Can you work these out from the model? Positions are in its coordinate system, mm. A direction names the side the tool comes from. Give positions to 0.01 mm unless a question says otherwise; leave off trailing zeros. Loops run counter-clockwise (first coordinate to the right, second up) from the corner with the lowest first, then second, coordinate; pieces in that order, holes last. Notation, with made-up numbers: (3, 64.25) -> (10, 64.25) arc R16 ccw to (10, 89.25) -> close; hole circle Ø10 at (51, 26). An arc over 180 degrees is marked (long way). Use CSV: the item, a comma, the result in double quotes.
from build123d import *

# Parameters (mm, degrees)
F0_R     = 31
F1_DEPTH = 10


# Not quite as in the source:
# - a feature names something its author has since deleted; it is built from what else it names


with BuildPart() as f1:
    # F0 (on Top) → F1 (new body)
    with BuildSketch(Plane.XY):
        Circle(F0_R)
        with BuildLine():
            ThreePointArc((19.2857142857, 8.310308327), (24.1116779802, 5.3418830281), (26, 0))
            ThreePointArc((26, 0), (24.1116779802, -5.3418830281), (19.2857142857, -8.310308327))
            ThreePointArc((19.2857142857, -8.310308327), (18.1865334795, -10.5), (16.8397952673, -12.5467643381))
            ThreePointArc((16.8397952673, -12.5467643381), (17.1468226066, -13.83507715), (17.25, -15.1554445662))
            ThreePointArc((17.25, -15.1554445662), (11.8049395785, -23.0874899627), (2.4459190184, -20.8570726651))
            ThreePointArc((2.4459190184, -20.8570726651), (0, -21), (-2.4459190184, -20.8570726651))
            ThreePointArc((-2.4459190184, -20.8570726651), (-13, -22.5166604984), (-16.8397952673, -12.5467643381))
            ThreePointArc((-16.8397952673, -12.5467643381), (-18.1865334795, -10.5), (-19.2857142857, -8.310308327))
            ThreePointArc((-19.2857142857, -8.310308327), (-26, 0), (-19.2857142857, 8.310308327))
            ThreePointArc((-19.2857142857, 8.310308327), (-18.1865334795, 10.5), (-16.8397952673, 12.5467643381))
            ThreePointArc((-16.8397952673, 12.5467643381), (-13, 22.5166604984), (-2.4459190184, 20.8570726651))
            ThreePointArc((-2.4459190184, 20.8570726651), (0, 21), (2.4459190184, 20.8570726651))
            ThreePointArc((2.4459190184, 20.8570726651), (11.8049395785, 23.0874899627), (17.25, 15.1554445662))
            ThreePointArc((17.25, 15.1554445662), (17.1468226066, 13.83507715), (16.8397952673, 12.5467643381))
            ThreePointArc((16.8397952673, 12.5467643381), (18.1865334795, 10.5), (19.2857142857, 8.310308327))
        make_face(mode=Mode.SUBTRACT)
    extrude(amount=F1_DEPTH)


solid = f1.part
(1) We'd pull the mould along X, two halves only. Please class faces 3 (the face through (-4.036, 30.736, 4.93)), 4 (the face through (-19, -11, 10)), 5 (the face through (-12.859, -22.596, 4.93)): released by +X, released by -X, zero draft, split by the parting line, or undercut.
Answer sheet:
face 3,"split by the parting line"
face 4,"zero draft"
face 5,"undercut"
(2) If we section it at D-D, the plane y = 25: Write out the boundary of the cut face in (x, z).
Answer sheet:
outline,"(-18.33, 0) -> (18.33, 0) -> (18.33, 10) -> (-18.33, 10) -> close"
(3) If we section it at C-C, the plane y = -1.5: Write out the boundary of the cut face in (x, z).
Answer sheet:
outline,"(-30.96, 0) -> (-25.87, 0) -> (-25.87, 10) -> (-30.96, 10) -> close; (25.87, 0) -> (30.96, 0) -> (30.96, 10) -> (25.87, 10) -> close"
(4) If we section it at A-A, the plane x = 0: Write out the boundary of the cut face in (y, z).
Answer sheet:
outline,"(-31, 0) -> (-21, 0) -> (-21, 10) -> (-31, 10) -> close; (21, 0) -> (31, 0) -> (31, 10) -> (21, 10) -> close"
(5) If I drill on L1, parallel to Y at x = 1, z = 5.5; L2, parallel to X at y = 22.5, z = 6.25; L3, parallel to Y at x = -9, z = 2.75, over which ranges is the centre line in solid material (lowest first)? Write a range as from..to.
Answer sheet:
L1,"y = -30.98..-20.98, 20.98..30.98"
L2,"x = -21.32..-13.03, -4.47..4.47, 13.03..21.32"
L3,"y = -29.66..-23.65, 23.65..29.66"
(6) Which directions (+Z, -Z, +X, -X, +Y, -Y) give clear straight access to the entire face, cutting with the end or side of a thin tool? Please do faces 1 (the face through (-19, -11, 0)), 2 (the face through (-26, 0, 5)).
Answer sheet:
face 1,"-Z, +X, -X, +Y, -Y"
face 2,"+Z, -Z"
(7) If we section it at B-B, the plane z = 9: Write out the boundary of the cut face in (x, y).
Answer sheet:
outline,"circle Ø62 at (0, 0); hole (-19.29, -8.31) arc R21 ccw to (-16.84, -12.55) arc R8.5 ccw to (-2.45, -20.86) arc R21 ccw to (2.45, -20.86) arc R8.5 ccw to (16.84, -12.55) arc R21 ccw to (19.29, -8.31) arc R8.5 ccw to (19.29, 8.31) arc R21 ccw to (16.84, 12.55) arc R8.5 ccw to (2.45, 20.86) arc R21 ccw to (-2.45, 20.86) arc R8.5 ccw to (-16.84, 12.55) arc R21 ccw to (-19.29, 8.31) arc R8.5 ccw to start"
(8) Will these pins go through, and if not, where does the flat tip stop? pin 1 Ø5 at (x, z) = (-19.5, 8) entering from -Y; pin 2 Ø1.5 at (x, y) = (-13, 20.5) entering from -Z; pin 3 Ø1.5 at (y, z) = (14, 4.5) entering from +X; pin 4 Ø6 at (x, z) = (14.5, 6) entering from -Y.
Answer sheet:
pin 1,"stops at y = -25.92"
pin 2,"passes through"
pin 3,"stops at x = 28.03"
pin 4,"stops at y = -28.79"
